Geometry check sheet. Reference: the model listing, model coordinates, mm. A direction names the side the tool comes from. Give positions to 0.01 mm unless a question says otherwise; leave off trailing zeros. Order: outer loops, then holes, each group sorted by start corner. A loop starts at its lowest first (then second) coordinate and runs counter-clockwise, first axis right, second up.
```python
from build123d import *

# Parameters (mm, degrees)
SKETCH_1_R      = 1
EXTRUDE_2_DEPTH = 3
SKETCH_3_R      = 1
EXTRUDE_3_DEPTH = 3
EXTRUDE_4_DEPTH = 3
EXTRUDE_5_DEPTH = 3
EXTRUDE_6_DEPTH = 3
CHAMFER_1_SIZE  = 0.25


with BuildPart() as part:
    # 草图1 → 凸台-拉伸2 (new body)
    with BuildSketch(Plane(origin=(0, 0, 0), x_dir=(1, 0, 0), z_dir=(0, 1, 0))):
        with BuildLine():
            Line((2, 1.5), (13, 1.5))
            ThreePointArc((13, 1.5), (15, 2.5), (17, 1.5))
            Line((17, 1.5), (63, 1.5))
            ThreePointArc((63, 1.5), (67.5, 0), (63, -1.5))
            Line((63, -1.5), (17, -1.5))
            ThreePointArc((17, -1.5), (15, -2.5), (13, -1.5))
            Line((13, -1.5), (2, -1.5))
            ThreePointArc((2, -1.5), (-2.5, 0), (2, 1.5))
        make_face()
        with Locations(Location((0, 0, 0), (0, 0, 270))):
            Circle(SKETCH_1_R, mode=Mode.SUBTRACT)
        with Locations(Location((15, 0, 0), (0, 0, 270))):
            Circle(SKETCH_1_R, mode=Mode.SUBTRACT)
        with Locations(Location((65, 0, 0), (0, 0, 270))):
            Circle(SKETCH_1_R, mode=Mode.SUBTRACT)
    extrude(amount=EXTRUDE_2_DEPTH)

    # 草图3 → 凸台-拉伸3 (add)
    with BuildSketch(Plane(origin=(0, 0, 0), x_dir=(1, 0, 0), z_dir=(0, 1, 0))):
        with BuildLine():
            Line((15.005676781, 2.499993555), (42.689167846, 39.237227017))
            ThreePointArc((42.689167846, 39.237227017), (46.595288715, 41.928364277), (45.085074376, 37.431781948))
            Line((45.085074376, 37.431781948), (17.401583311, 0.694548485))
            ThreePointArc((17.401583311, 0.694548485), (17.440740018, 0.541099035), (17.47010253, 0.385478264))
            Line((17.47010253, 0.385478264), (58.085691801, -21.210213624))
            ThreePointArc((58.085691801, -21.210213624), (61.354748625, -24.647257046), (56.677277113, -23.859056403))
            Line((56.677277113, -23.859056403), (16.061687842, -2.263364515))
            ThreePointArc((16.061687842, -2.263364515), (12.559259982, -0.541099035), (15.005676781, 2.499993555))
        make_face()
        with Locations(Location((59.147379643, -23.473578139, 0), (0, 0, 270))):
            Circle(SKETCH_3_R, mode=Mode.SUBTRACT)
        with Locations(Location((45.090751158, 39.931775502, 0), (0, 0, 270))):
            Circle(SKETCH_3_R, mode=Mode.SUBTRACT)
        with Locations(Location((15, 0, 0), (0, 0, 270))):
            Circle(SKETCH_3_R, mode=Mode.SUBTRACT)
    extrude(amount=EXTRUDE_3_DEPTH)

    # 草图5 → 凸台-拉伸4 (add)
    with BuildSketch(Plane(origin=(0, 0, 0), x_dir=(1, 0, 0), z_dir=(0, 1, 0))):
        Polygon((50.968736425, 1.5), (37.844479209, 27.823187626), (39.651372694, 30.221016268), (53.97114317, 1.5), align=None)
    extrude(amount=EXTRUDE_4_DEPTH)

    # 草图6 → 凸台-拉伸5 (add)
    with BuildSketch(Plane(origin=(0, 0, 0), x_dir=(1, 0, 0), z_dir=(0, 1, 0))):
        Polygon((54.971865105, -1.5), (50.997269421, -17.441232589), (53.647846432, -18.850569385), (57.973829245, -1.5), align=None)
    extrude(amount=EXTRUDE_5_DEPTH)

    # 草图7 → 凸台-拉伸6 (add)
    with BuildSketch(Plane(origin=(0, 0, 0), x_dir=(1, 0, 0), z_dir=(0, 1, 0))):
        with BuildLine():
            Line((4.5, 1.5), (0.578145188, 2.432231104))
            ThreePointArc((0.578145188, 2.432231104), (1.370755945, 2.090700395), (2, 1.5))
            Line((2, 1.5), (4.5, 1.5))
        make_face()
        with BuildLine():
            Line((4.5, -1.5), (0.578145188, -2.432231104))
            ThreePointArc((0.578145188, -2.432231104), (1.370755945, -2.090700395), (2, -1.5))
            Line((2, -1.5), (4.5, -1.5))
        make_face()
        with BuildLine():
            Line((10.5, 1.5), (14.421854812, 2.432231104))
            ThreePointArc((14.421854812, 2.432231104), (13.629244055, 2.090700395), (13, 1.5))
            Line((13, 1.5), (10.5, 1.5))
        make_face()
        with BuildLine():
            Line((10.5, -1.5), (14.421854812, -2.432231104))
            ThreePointArc((14.421854812, -2.432231104), (13.629244055, -2.090700395), (13, -1.5))
            Line((13, -1.5), (10.5, -1.5))
        make_face()
        with BuildLine():
            Line((41.184630288, 37.240638242), (42.80034857, 40.933801444))
            ThreePointArc((42.80034857, 40.933801444), (42.596102061, 40.095256036), (42.689167846, 39.237227017))
            Line((42.689167846, 39.237227017), (41.184630288, 37.240638242))
        make_face()
        with BuildLine():
            Line((43.580536818, 35.435193172), (46.685280826, 38.006295008))
            ThreePointArc((46.685280826, 38.006295008), (45.935517213, 37.578826223), (45.085074376, 37.431781948))
            Line((45.085074376, 37.431781948), (43.580536818, 35.435193172))
        make_face()
        with BuildLine():
            Line((60.5, -1.5), (64.421854812, -2.432231104))
            ThreePointArc((64.421854812, -2.432231104), (63.629244055, -2.090700395), (63, -1.5))
            Line((63, -1.5), (60.5, -1.5))
        make_face()
        with BuildLine():
            Line((60.5, 1.5), (64.421854812, 2.432231104))
            ThreePointArc((64.421854812, 2.432231104), (63.629244055, 2.090700395), (63, 1.5))
            Line((63, 1.5), (60.5, 1.5))
        make_face()
        with BuildLine():
            Line((55.878322819, -20.036534717), (59.778771079, -21.054622816))
            ThreePointArc((59.778771079, -21.054622816), (58.918598363, -20.984068323), (58.085691801, -21.210213624))
            Line((58.085691801, -21.210213624), (55.878322819, -20.036534717))
        make_face()
        with BuildLine():
            Line((54.469908131, -22.685377496), (57.495044404, -25.349688013))
            ThreePointArc((57.495044404, -25.349688013), (56.9555496, -24.676026085), (56.677277113, -23.859056403))
            Line((56.677277113, -23.859056403), (54.469908131, -22.685377496))
        make_face()
    extrude(amount=EXTRUDE_6_DEPTH)

    # 倒角1
    chamfer_1_edges = [part.edges().sort_by_distance(p)[0] for p in [
        (57.235571585, 0, -1.5),
        (57.235571585, 3, -1.5),
        (62.460927406, 0, -1.966115552),
        (62.460927406, 3, -1.966115552),
        (46.595288715, 3, -41.928364277),
        (46.595288715, 0, -41.928364277),
        (45.132908822, 0, -36.72074409),
        (45.132908822, 3, -36.72074409),
        (-2.5, 0, 0),
        (-2.5, 3, 0),
        (2.539072594, 0, -1.966115552),
        (2.539072594, 3, -1.966115552),
        (28.095153535, 3, -19.870315898),
        (28.095153535, 0, -19.870315898),
        (41.992489429, 0, -39.087219843),
        (41.992489429, 3, -39.087219843),
        (7.5, 0, 1.5),
        (7.5, 3, 1.5),
        (2.539072594, 0, 1.966115552),
        (2.539072594, 3, 1.966115552),
        (7.5, 0, -1.5),
        (7.5, 3, -1.5),
        (12.460927406, 0, -1.966115552),
        (12.460927406, 3, -1.966115552),
        (15.256090523, 0, 2.486848939),
        (15.256090523, 3, 2.486848939),
        (12.460927406, 0, 1.966115552),
        (12.460927406, 3, 1.966115552),
        (61.354748625, 3, 24.647257046),
        (61.354748625, 0, 24.647257046),
        (55.982476267, 0, 24.017532754),
        (55.982476267, 3, 24.017532754),
        (54.763084626, 0, 19.443552051),
        (54.763084626, 3, 19.443552051),
        (57.828546949, 0, 20.545578767),
        (57.828546949, 3, 20.545578767),
        (67.5, 0, 0),
        (67.5, 3, 0),
        (62.460927406, 0, 1.966115552),
        (62.460927406, 3, 1.966115552),
        (0, 0, -1),
        (0, 3, -1),
        (15, 0, -1),
        (15, 3, -1),
        (65, 0, -1),
        (65, 3, -1),
        (14.71176753, 0, -2.483328823),
        (14.71176753, 3, -2.483328823),
        (37.994018253, 0, 1.5),
        (37.994018253, 3, 1.5),
        (27.926506886, 0, -14.661593813),
        (59.147379643, 0, 22.473578139),
        (45.090751158, 0, -40.931775502),
        (35.265797986, 3, 12.474371005),
        (27.926506886, 3, -14.661593813),
        (45.090751158, 3, -40.931775502),
        (59.147379643, 3, 22.473578139),
        (35.265797986, 0, 12.474371005),
        (41.615954756, 3, -32.82810472),
        (41.615954756, 0, -32.82810472),
        (34.488635494, 0, -1.5),
        (34.488635494, 3, -1.5),
        (46.811257932, 0, -15.860508134),
        (44.406607817, 0, -14.661593813),
        (44.406607817, 3, -14.661593813),
        (46.811257932, 3, -15.860508134),
        (36.006720411, 0, 9.470616295),
        (36.006720411, 3, 9.470616295),
        (59.236914623, 0, 1.5),
        (59.236914623, 3, 1.5),
        (55.810837839, 0, 10.175284693),
        (52.984567263, 0, 9.470616295),
        (52.984567263, 3, 9.470616295),
        (55.810837839, 3, 10.175284693),
    ]]
    chamfer(chamfer_1_edges, length=CHAMFER_1_SIZE)


solid = part.part
```
Q1. Cross-section at A-A, the plane z = 0. Give the number of separate pieces and of enclosed holes in the cut face, and give its area (4 significant figures).
Q2. Release check for a two-part mould opening along X. For faces 1 (the face through (45.11, 1.48, -36.7)), 2 (the face through (35.43, 2.87, 9.3)), 3 (the face through (42, 1.5, -39.1)), 4 (the face through (46.47, 0.13, -41.87)) record: pulls with the +X half, pulls with the -X half, needs draft (parallel to the pull), parting line crosses it, or undercut.
Q3. Cross-section at B-B, the plane z = 16.5. Record the boundary of the cut face in (x, y), and give its area (3 significant figures).
Q4. Cross-section at C-C, the plane z = -7. Record the boundary of the cut face in (x, y).
Q5. Access from +Z, -Z, +X, -X, +Y, -Y to the whole of each face (thin tool, end or side, straight path). Record for faces 5 (the face through (53.13, 2.87, 9.38)), 6 (the face through (34, 1, -1.5)), 7 (the face through (44.611, 0.127, -14.527)), 8 (the face through (42.088, 0.127, -38.998)).
Q6. Thickness scan on L1, parallel to Z at x = 41.5, y = 1.95; L2, parallel to X at y = 1.65, z = 0; L3, parallel to Z at x = 10, y = 0.95. Record the ranges inside material, lowest first.
Q7. Gauge pin test, flat end, axial feed: P1, Ø1.8, axis at x = 45.09, z = -39.93, coming from the -Y side. Record the tip position at first contact, or that the pin passes through.
Answers follow:
1. separate pieces: 4
1. enclosed holes: 0
1. area: 191.5 mm2
2. face 1: pulls with the +X half
2. face 2: undercut
2. face 3: pulls with the -X half
2. face 4: parting line crosses it
3. outline: (42.84, 0.25) - (43.37, 0) - (48.69, 0) - (49.23, 0.25) - (49.23, 2.75) - (48.69, 3) - (43.37, 3) - (42.84, 2.75) - close; (51.23, 0.25) - (51.49, 0) - (53.98, 0) - (54.23, 0.25) - (54.23, 2.75) - (53.98, 3) - (51.49, 3) - (51.23, 2.75) - close
3. area: 27.8 mm2
4. outline: (18.4, 0.25) - (18.71, 0) - (21.84, 0) - (22.15, 0.25) - (22.15, 2.75) - (21.84, 3) - (18.71, 3) - (18.4, 2.75) - close; (48.23, 0.25) - (48.51, 0) - (50.95, 0) - (51.23, 0.25) - (51.23, 2.75) - (50.95, 3) - (48.51, 3) - (48.23, 2.75) - close
5. face 5: +Y
5. face 6: +Y, -Y
5. face 7: -Y
5. face 8: -Z, -X, -Y
6. L1: z = -37.96 to -32.67, -26.51 to -20.49, -1.5 to 1.5, 12.39 to 15.79
6. L2: x = -2.5 to -1, 1 to 14, 16 to 64, 66 to 67.5
6. L3: z = -1.5 to 1.5
7. P1: passes through
